Geometry check sheet. Reference: the model listing, model coordinates, mm. A direction names the side the tool comes from. Coordinates: 2 decimals unless noted, no trailing zeros. Write each loop counter-clockwise with the first axis right and the second up, starting at its lowest first coordinate (ties: lowest second). Pieces come first, ordered by that corner, then holes. Notation, with made-up numbers: (4, 77) -> (26, 77) arc R26 cw to (26, 114) -> close; hole circle Ø1 at (-26, 31.5). An arc over 180 degrees is marked (long way). Answer as CSV lines item,"result".
```python
from build123d import *

# Parameters (mm, degrees)
SKETCH_8_W               = 96
SKETCH_8_H               = 96
SKETCH_8_R               = 43.9
EXTRUDE_1_DEPTH          = 33.54
CUT_EXTRUDE_3_DEPTH      = 84.429752707
CUT_EXTRUDE_3_DEPTH_BACK = 8.53
SKETCH_14_W              = 6
SKETCH_14_H              = 96
EXTRUDE_3_DEPTH          = 18.502821
EXTRUDE_3_DEPTH_BACK     = 14
SKETCH_16_W              = 22.4
SKETCH_16_H              = 4
SKETCH_16_W_2            = 7.4
SKETCH_16_H_2            = 22
SKETCH_16_R              = 2.5
FILLET_5_R               = 4
SKETCH_21_W              = 30.907014898
SKETCH_21_H              = 30.907014898
SKETCH_21_R              = 11
EXTRUDE_4_DEPTH          = 4
SKETCH_22_R              = 2.5
CUT_EXTRUDE_4_DEPTH      = 87.584546233
CUT_EXTRUDE_5_DEPTH      = 125.935517954
CUT_EXTRUDE_5_DEPTH_BACK = 125.935517954
SKETCH_23_W              = 6
SKETCH_23_H              = 8


with BuildPart() as part:
    # 掃出1: sweep along a path in 草圖6
    with BuildLine(Plane(origin=(0, 0, 0), x_dir=(1, 0, 0), z_dir=(0, 1, 0))) as sweep_1_path:
        Line((-42, 42), (42, 42))
        Line((42, 42), (42, -42))
        Line((42, -42), (-42, -42))
        Line((-42, -42), (-42, 42))
    # 草圖7 → 掃出1 (sweep)
    with BuildSketch(Plane.XY):
        with BuildLine():
            Line((-48, 0), (-48, 14.962820915))
            Line((-48, 14.962820915), (-41.427728365, 14.962820915))
            Line((-41.427728365, 14.962820915), (-41.427728365, 5.074548504))
            Line((-41.427728365, 5.074548504), (-33.350791498, 5.074548504))
            Line((-33.350791498, 5.074548504), (-15.453507449, 15))
            Line((-15.453507449, 15), (-11, 15))
            add(Edge.make_bspline(
                [(-11, 15), (-19.96241049, 7.783643124), (-30.446618789, 1.65287244), (-42, 0)],
                knots=[0, 0, 0, 0, 1, 1, 1, 1], degree=3))
            Line((-42, 0), (-48, 0))
        make_face()
    sweep(path=sweep_1_path.line, transition=Transition.RIGHT)

    # 草圖8 → 填料-伸長1 (add)
    with BuildSketch(Plane(origin=(0, 14.962820915, 0), x_dir=(1, 0, 0), z_dir=(0, 1, 0))):
        Rectangle(SKETCH_8_W, SKETCH_8_H)
        with Locations(Location((0, 0, 0), (0, 0, 70.679739301))):
            Circle(SKETCH_8_R, mode=Mode.SUBTRACT)
    extrude(amount=EXTRUDE_1_DEPTH)

    # 草圖14 → 除料-伸長3 (cut, two sides: drawn at the far end of the back side and taken through both)
    with BuildSketch(Plane(origin=(0, 0, 0), x_dir=(1, 0, 0), z_dir=(0, 1, 0)).offset(-CUT_EXTRUDE_3_DEPTH_BACK)):
        with Locations((-45, 0)):
            Rectangle(SKETCH_14_W, SKETCH_14_H)
    extrude(amount=CUT_EXTRUDE_3_DEPTH + CUT_EXTRUDE_3_DEPTH_BACK, mode=Mode.SUBTRACT)

    # 草圖16 → 填料-伸長3 (add, two sides: drawn at the far end of the back side and taken through both)
    # profile 1 of 4: a face of its own
    with BuildSketch(Plane(origin=(0, 30, 0), x_dir=(1, 0, 0), z_dir=(0, 1, 0)).offset(-EXTRUDE_3_DEPTH_BACK)):
        with Locations((36.8, 50)):
            Rectangle(SKETCH_16_W, SKETCH_16_H)
    # profile 2 of 4: a face of its own
    with BuildSketch(Plane(origin=(0, 30, 0), x_dir=(1, 0, 0), z_dir=(0, 1, 0)).offset(-EXTRUDE_3_DEPTH_BACK)):
        with Locations((36.8, -50)):
            Rectangle(SKETCH_16_W, SKETCH_16_H)
    # profile 3 of 4: a face of its own
    with BuildSketch(Plane(origin=(0, 30, 0), x_dir=(1, 0, 0), z_dir=(0, 1, 0)).offset(-EXTRUDE_3_DEPTH_BACK)):
        with Locations((-45.7, -37)):
            Rectangle(SKETCH_16_W_2, SKETCH_16_H_2)
        with Locations(Location((-45, -37, 0), (0, 0, 270))):
            Circle(SKETCH_16_R, mode=Mode.SUBTRACT)
    # profile 4 of 4: a face of its own
    with BuildSketch(Plane(origin=(0, 30, 0), x_dir=(1, 0, 0), z_dir=(0, 1, 0)).offset(-EXTRUDE_3_DEPTH_BACK)):
        with Locations((-45.7, 37)):
            Rectangle(SKETCH_16_W_2, SKETCH_16_H_2)
        with Locations(Location((-45, 37, 0), (0, 0, 270))):
            Circle(SKETCH_16_R, mode=Mode.SUBTRACT)
    extrude(amount=EXTRUDE_3_DEPTH + EXTRUDE_3_DEPTH_BACK)

    # 圓角5
    fillet_5_edges = [part.edges().sort_by_distance(p)[0] for p in [
        (3, 0, -48),
        (48, 0, 0),
        (3, 0, 48),
    ]]
    fillet(fillet_5_edges, radius=FILLET_5_R)

    # 草圖21 → 填料-伸長4 (add)
    with BuildSketch(Plane(origin=(0, 15, 0), x_dir=(1, 0, 0), z_dir=(0, 1, 0))):
        Rectangle(SKETCH_21_W, SKETCH_21_H)
        with Locations(Location((0, 0, 0), (0, 0, 270))):
            Circle(SKETCH_21_R, mode=Mode.SUBTRACT)
    extrude(amount=EXTRUDE_4_DEPTH)

    # 草圖22 → 除料-伸長4 (cut, through all)
    with BuildSketch(Plane(origin=(0, 48.502820915, 0), x_dir=(1, 0, 0), z_dir=(0, 1, 0))):
        with Locations(Location((36.142689786, 47.122458141, 0), (0, 0, 270))):
            Circle(SKETCH_22_R)
        with Locations(Location((36.142689786, -47.122458141, 0), (0, 0, 339.450483695))):
            Circle(SKETCH_22_R)
    extrude(amount=-CUT_EXTRUDE_4_DEPTH, mode=Mode.SUBTRACT)

    # 草圖23 → 除料-伸長5 (cut, two sides: drawn at the far end of the back side and taken through both)
    with BuildSketch(Plane(origin=(0, 0, -52), x_dir=(-1, 0, 0), z_dir=(0, 0, -1)).offset(-CUT_EXTRUDE_5_DEPTH_BACK)):
        with Locations((-45, 10)):
            Rectangle(SKETCH_23_W, SKETCH_23_H)
    extrude(amount=CUT_EXTRUDE_5_DEPTH + CUT_EXTRUDE_5_DEPTH_BACK, mode=Mode.SUBTRACT)


solid = part.part
```
Item 1: Release check for a two-part mould opening along Y. For faces 1 (the flat face through (0, 14.963, -42)), 2 (the flat face through (41.428, 10, 1)), 3 (the flat face through (37, 16, 50)), 4 (the flat face through (37, 32, -52)) record: +Y half, -Y half, draft (parallel to the pull), parting line (faces both ways), or undercut.
Responses:
face 1,"+Y half"
face 2,"undercut"
face 3,"-Y half"
face 4,"draft"
Item 2: Cross-section at B-B, the plane y = 37. Record the cut outline in (x, z).
Responses:
outline,"(-49.4, -48) -> (25.6, -48) -> (25.6, -52) -> (48, -52) -> (48, 52) -> (25.6, 52) -> (25.6, 48) -> (-49.4, 48) -> (-49.4, 26) -> (-42, 26) -> (-42, 12.78) arc R43.9 cw (long way) to (-42, -12.78) -> (-42, -26) -> (-49.4, -26) -> close; hole circle Ø5 at (-45, -37); hole circle Ø5 at (-45, 37); hole circle Ø5 at (36.14, -47.12); hole circle Ø5 at (36.14, 47.12)"
Item 3: Cross-section at A-A, the plane x = -45. Record the cut outline in (y, z).
Responses:
outline,"(16, -48) -> (48.5, -48) -> (48.5, -39.5) -> (16, -39.5) -> close; (16, -34.5) -> (48.5, -34.5) -> (48.5, -26) -> (16, -26) -> close; (16, 26) -> (48.5, 26) -> (48.5, 34.5) -> (16, 34.5) -> close; (16, 39.5) -> (48.5, 39.5) -> (48.5, 48) -> (16, 48) -> close"
Item 4: Thickness scan on probe 1 along Z at (x, y) = (0, 17.35); probe 2 along X at (y, z) = (19.5, -47.5); probe 3 along X at (y, z) = (33, 47). Record the ranges inside material, lowest first.
Responses:
probe 1,"z = -48 to -43.9, -15.45 to -11, 11 to 15.45, 43.9 to 48"
probe 2,"x = -49.4 to 33.67, 38.61 to 48"
probe 3,"x = -49.4 to 33.65, 38.64 to 48"
Item 5: Depth check by flat-ended pin: pin 1 Ø3 at (x, z) = (37, -51) entering from -Y; pin 2 Ø2 at (x, y) = (-45.5, 38) entering from +Z; pin 3 Ø12 at (x, z) = (6.5, 3.5) entering from -Y. Enter the tip coordinate at first touch or a pass-through.
Responses:
pin 1,"stops at y = 16"
pin 2,"stops at z = 48"
pin 3,"stops at y = 13.81"
Item 6: Set-up check for faces 5 (the flat face through (-46, 16, 34)), 6 (the flat face through (-41.428, 10, -1)), 7 (the flat face through (25.6, 32, 50)), 8 (the flat face through (-46, 32, -26)), 9 (the flat face through (-9, 15, 8)): record each of +Z, -Z, +X, -X, +Y, -Y from which the full face is reachable in a straight line by a thin tool's end or side.
Responses:
face 5,"+Z, -Z, -X, -Y"
face 6,"none"
face 7,"+Z, -X, +Y, -Y"
face 8,"-X, +Y, -Y"
face 9,"-Y"
